from build123d import *

# Parameters (mm, degrees)
SKETCH1_W           = 100
SKETCH1_H           = 50
BOSS_EXTRUDE2_DEPTH = 10
SKETCH3_W           = 80
SKETCH3_H           = 50
BOSS_EXTRUDE3_DEPTH = 10
SKETCH4_W           = 40
SKETCH4_H           = 50
BOSS_EXTRUDE4_DEPTH = 25
SKETCH5_W           = 60
SKETCH5_H           = 30
CUT_EXTRUDE1_DEPTH  = 25
SKETCH6_R           = 15
SKETCH6_R_2         = 12
BOSS_EXTRUDE5_DEPTH = 5
CHAMFER2_SIZE       = 10
CHAMFER3_SIZE       = 10
FILLET3_R           = 2
CHAMFER6_SIZE       = 27.5


# Some blends are built 0.0001 mm under size
with BuildPart() as part:
    # Sketch1 → Boss-Extrude2 (new body)
    with BuildSketch(Plane.XY):
        Rectangle(SKETCH1_W, SKETCH1_H)
    extrude(amount=BOSS_EXTRUDE2_DEPTH)

    # Sketch3 → Boss-Extrude3 (add)
    with BuildSketch(Plane.XY.offset(10)):
        Rectangle(SKETCH3_W, SKETCH3_H)
    extrude(amount=BOSS_EXTRUDE3_DEPTH)

    # Sketch4 → Boss-Extrude4 (add)
    with BuildSketch(Plane.XY.offset(20)):
        with Locations((-20, 0)):
            Rectangle(SKETCH4_W, SKETCH4_H)
    extrude(amount=BOSS_EXTRUDE4_DEPTH)

    # Sketch5 → Cut-Extrude1 (cut)
    with BuildSketch(Plane.XY.offset(45)):
        with Locations((2.565042783, 0)):
            Rectangle(SKETCH5_W, SKETCH5_H)
    extrude(amount=-CUT_EXTRUDE1_DEPTH, mode=Mode.SUBTRACT)

    # Sketch6 → Boss-Extrude5 (add)
    with BuildSketch(Plane.XY.offset(20)):
        with Locations((15, 0)):
            Circle(SKETCH6_R)
        with Locations((15, 0)):
            Circle(SKETCH6_R_2, mode=Mode.SUBTRACT)
    extrude(amount=BOSS_EXTRUDE5_DEPTH)

    # Chamfer2
    chamfer2_edges = [part.edges().sort_by_distance(p)[0] for p in [
        (50, 0, 10),
    ]]
    chamfer(chamfer2_edges, length=CHAMFER2_SIZE - 0.0001)  # a hair under: the kernel refuses the full size

    # Chamfer3
    chamfer3_edges = [part.edges().sort_by_distance(p)[0] for p in [
        (-50, 0, 10),
    ]]
    chamfer(chamfer3_edges, length=CHAMFER3_SIZE - 0.0001)  # a hair under: the kernel refuses the full size

    # Fillet3
    fillet3_edges = [part.edges().sort_by_distance(p)[0] for p in [
        (0, 0, 20),
    ]]
    fillet(fillet3_edges, radius=FILLET3_R)

    # Chamfer6
    # the kernel refuses this chamfer: 27.5 mm, written as the material it takes off along each edge
    with BuildSketch(Plane(origin=(0, -15, 45), x_dir=(0.027495876610586376, 0, -0.9996219169112968), z_dir=(0, -1, 0))) as chamfer6_piece_1_section:
        Polygon((CHAMFER6_SIZE * 0.999621916911, -CHAMFER6_SIZE * 0.0274958766106), (-CHAMFER6_SIZE * 0.0274958766106, -CHAMFER6_SIZE * 0.999621916911), (0, 0), align=None)
    chamfer6_piece_1 = extrude(amount=80.721282169, mode=Mode.PRIVATE)
    chamfer6_piece_1 = split(chamfer6_piece_1, bisect_by=Plane(origin=(-2.708333333, -20, 20), z_dir=(0, 0, 1)), keep=Keep.TOP, mode=Mode.PRIVATE)
    add(chamfer6_piece_1, mode=Mode.SUBTRACT)
    with BuildSketch(Plane(origin=(0, 55.721282169, 45), x_dir=(0.027495876610586376, 0, -0.9996219169112968), z_dir=(0, -1, 0))) as chamfer6_piece_2_section:
        Polygon((CHAMFER6_SIZE * 0.999621916911, -CHAMFER6_SIZE * 0.0274958766106), (-CHAMFER6_SIZE * 0.0274958766106, -CHAMFER6_SIZE * 0.999621916911), (0, 0), align=None)
    chamfer6_piece_2 = extrude(amount=151.442564338, mode=Mode.PRIVATE)
    chamfer6_piece_2 = split(chamfer6_piece_2, bisect_by=Plane(origin=(-27.456638145, 15, 44.978319072), z_dir=(0, -1, 0)), keep=Keep.TOP, mode=Mode.PRIVATE)
    chamfer6_piece_2 = split(chamfer6_piece_2, bisect_by=Plane(origin=(-27.456638145, 0, 25), z_dir=(0, 0, 1)), keep=Keep.TOP, mode=Mode.PRIVATE)
    add(chamfer6_piece_2, mode=Mode.SUBTRACT)


solid = part.part
Check sheet for the modelled part. Datum: model origin and axes. Units: mm. A direction names the side the tool comes from. Give positions to 0.01 mm unless a question says otherwise; leave off trailing zeros. Order: outer loops, then holes, each group sorted by start corner. A loop starts at its lowest first (then second) coordinate and runs counter-clockwise, first axis right, second up. Notation, with made-up numbers: (78.5, 20) - (111.5, 20) arc R35 cw to (111.5, 59) - close; hole circle Ø2 at (2.25, 52). An arc over 180 degrees is marked (long way). Answer as CSV lines item,"result".
1. Section check A-A (z = 41). Record the boundary of the cut face in (x, y).
Result sheet:
outline,"(-40, -25) - (-23.5, -25) - (-23.5, -15) - (-27.43, -15) - (-27.43, 15) - (0, 15) - (0, 25) - (-40, 25) - close"
2. Go/stop test with flat-tipped pins: P1, Ø15, axis at x = 19.5, y = 4.5, coming from the +Z side; P2, Ø5, axis at y = 19.5, z = 38, coming from the +X side; P3, Ø1.5, axis at y = 14.5, z = 15.5, coming from the +X side. Record where each tip stops, or that it passes through.
Result sheet:
P1,"z = 25"
P2,"x = 0"
P3,"x = 40"
3. Section check C-C (x = -9.5). Record the boundary of the cut face in (y, z), then the cut area to 3 significant figures.
Result sheet:
outline,"(-25, 0) - (25, 0) - (25, 45) - (15, 45) - (15, 20) - (-15, 20) - (-15, 27) - (-25, 27) - close"
area,"1,320 mm²"
4. Mould release check, pull along Y, two halves, no side actions. Record for faces 1 (the face through (40, 0, 15)), 2 (the face through (-12, 25, 17)), 3 (the face through (-2, -5, 20)): released by +Y, released by -Y, zero draft, split by the parting line, or undercut.
Result sheet:
face 1,"zero draft"
face 2,"released by +Y"
face 3,"undercut"
5. Scan lines: probe 1 along Y at (x, z) = (15, 22); probe 2 along X at (y, z) = (-17, 12.5); probe 3 along Y at (x, z) = (15, 21.3). Record each from-to range of solid material in increasing order. Write a range as from..to.
Result sheet:
probe 1,"-15..-12, 12..15"
probe 2,"-40..40"
probe 3,"-15.13..-12, 12..15.13"
6. Tool access check on faces 4 (the face through (8, 10, 25)), 5 (the face through (3.01, 0.53, 22.46)), 6 (the face through (-40, 0, 27)). Record the directions out of +Z, -Z, +X, -X, +Y, -Y that give a thin tool (end or side, any length) a straight path to the whole face; none if there is none.
Result sheet:
face 4,"+Z, +X, +Y, -Y"
face 5,"+Z"
face 6,"+Z, -X, +Y, -Y"
